Autodesk Inventor part; units mm, degrees
ref_plane "YZ Plane" through (0, 0, 0) normal (1, 0, 0) x (0, 1, 0)
ref_plane "XZ Plane" through (0, 0, 0) normal (0, 1, 0) x (-1, 0, 0)
ref_plane "XY Plane" through (0, 0, 0) normal (0, 0, 1) x (1, 0, 0)
sketch "Sketch1" plane through (0, 0, 0) normal (0, 1, 0) x (-1, 0, 0)
  line L0 (29.21, 0) -> (29.21, 12.8)
  line L1 (29.21, 12.8) -> (0, 12.8)
  line L2 (29.21, 12.8) -> (13.21, 12.8)
  circle A0 centre (3.3025, 9.6) radius 1.5
  circle A1 centre (9.9075, 9.6) radius 1.5
  line L3 (0, 12.8) -> (0, 0)
  line L4 (0, 0) -> (29.21, 0)
  dimension "d0" = 12.8
  dimension "d1" = 16
  dimension "d4" = 3
  dimension "d5" = 3
extrude "Extrusion1" add sketch "Sketch1" along normal blind 3
sketch "Sketch2" plane through (0, 3, 0) normal (0, 1, 0) x (1, 0, 0)
  line L0 (0, 0) -> (-29.21, 0)
  line L1 (-29.21, -12.8) -> (0, -12.8)
  line L2 (-29.21, 0) -> (-26.21, 0)
  line L3 (-26.21, 0) -> (-26.21, -12.8)
  line L4 (-26.21, -12.8) -> (-29.21, -12.8)
  line L5 (-29.21, -12.8) -> (-29.21, 0)
  dimension "d8" = 3
extrude "Extrusion2" add sketch "Sketch2" along normal blind 29.2
sketch "Sketch3" plane through (-29.21, 0, 0) normal (-1, 0, 0) x (0, 0, 1)
  line L0 (12.8, 0) -> (12.8, 32.2)
  line L1 (12.8, 16.1) -> (0, 16.1)
  line L2 (0, 0) -> (0, 32.2)
  line L3 (6.4, 27.2) -> (12.3, 27.2)
  line L4 (12.3, 27.2) -> (12.3, 5)
  line L5 (12.3, 5) -> (0.5, 5)
  line L6 (0.5, 5) -> (0.5, 27.2)
  line L7 (0.5, 27.2) -> (6.4, 27.2)
  line L8 (0, 0) -> (12.8, 0)
  circle A0 centre (6.4, 2.5) radius 0.5
  line L9 (0, 32.2) -> (12.8, 32.2)
  circle A1 centre (6.4, 29.7) radius 0.5
  dimension "d12" = 5.9
  dimension "d13" = 11.8
  dimension "d14" = 1
  dimension "d15" = 1
extrude "Extrusion3" cut sketch "Sketch3" against normal blind 3 contours L4 L5 L6 L1 | L1 L6 L7 L3 L4 | A0 | A1
sketch "Эскиз5" plane through (0, 0, 0) normal (0, 0, -1) x (-1, 0, 0)
  line L0 (29.21, 0) -> (0, 0)
  line L1 (26.21, 32.2) -> (29.21, 32.2)
  line L2 (0, 0) -> (29.21, 0)
  line L3 (29.21, 0) -> (29.21, 32.2)
  line L4 (29.21, 32.2) -> (0, 32.2)
  line L5 (0, 32.2) -> (0, 0)
extrude "Выдавливание4" add sketch "Эскиз5" along normal blind 3
chamfer "Фаска1" distance 15 angle 45 1 edges at (0, 32.2, -1.5)
fillet "Сопряжение3" radius 3 2 edges at (0, 1.5, 12.8) (-27.71, 32.2, 12.8)
Verification items for the finished model (mm, model axes). A direction names the side the tool comes from. Round coordinates to 2 decimals unless told otherwise and drop trailing zeros. Order: outer loops, then holes, each group sorted by start corner. A loop starts at its lowest first (then second) coordinate and runs counter-clockwise, first axis right, second up. Notation, with made-up numbers: (-5, 56) - (36, 56) arc R13 cw to (36, 72) - close; hole circle Ø9 at (-30.5, -28). An arc over 180 degrees is marked (long way). Use CSV: the item, a comma, the result in double quotes. Start each with the question number.
1) Thickness scan on L1, parallel to Y at x = -28.4, z = 6.4; L2, parallel to Y at x = -27, z = 8.75; L3, parallel to Z at x = -8.25, y = 4. Record the ranges inside material, lowest first.
2) Go/stop test with flat-tipped pins: P1, Ø2, axis at x = -20, y = 9.5, coming from the +Z side; P2, Ø1.8, axis at x = -9.91, z = 9.6, coming from the +Y side; P3, Ø1, axis at y = 18, z = -1, coming from the +X side. Record where each tip stops, or that it passes through.
3) Section check A-A, the plane y = 23. Record the cut outline in (x, z), plus the area to 3 significant figures.
4) Access from +Z, -Z, +X, -X, +Y, -Y to the whole of each face (thin tool, end or side, straight path). Record for faces 1 (the flat face through (-26.21, 20.8, 0.2)), 2 (the flat face through (-28, 5, 6)), 3 (the flat face through (-26.21, 2.5, 6.4)), 4 (the cylindrical face through (-27.69, 31.34, 11.9)).
5) Mould release check, pull along Y, two halves, no side actions. Record for faces 5 (the flat face through (-14, 16, -3)), 6 (the cylindrical face through (-27.731, 2.65, 6.877)), 7 (the flat face through (-15, 0, 5)), 8 (the flat face through (-28, 16, 12.3)): +Y half, -Y half, draft (parallel to the pull), parting line (faces both ways), or undercut.
6) Section check C-C, the plane y = 2.5. Record the cut outline in (x, z), plus the area to 3 significant figures.
7) Section check B-B, the plane z = 3. Record the cut outline in (x, y), plus the area to 3 significant figures.
8) Section check D-D, the plane x = -24.75. Record the cut outline in (y, z), plus the area to 3 significant figures.
Answers:
1,L1,"y = 0 to 2, 3 to 5, 27.2 to 29.2, 30.2 to 32.2"
1,L2,"y = 0 to 5, 27.2 to 32.2"
1,L3,"z = -3 to 0"
2,P1,"stops at z = 0"
2,P2,"passes through"
2,P3,"stops at x = -0.3"
3,outline,"(-29.21, -3) - (-5.8, -3) - (-5.8, 0) - (-26.21, 0) - (-26.21, 0.5) - (-29.21, 0.5) - close; (-29.21, 12.3) - (-26.21, 12.3) - (-26.21, 12.8) - (-29.21, 12.8) - close"
3,area,"73.2 mm²"
4,face 1,"+Z, +X, +Y"
4,face 2,"+X, -X"
4,face 3,"-X"
4,face 4,"+Z, +X, -X, +Y"
5,face 5,"draft"
5,face 6,"undercut"
5,face 7,"-Y half"
5,face 8,"undercut"
6,outline,"(-29.21, -3) - (0, -3) - (0, 9.8) arc R3 ccw to (-3, 12.8) - (-29.21, 12.8) - (-29.21, 6.9) - (-26.21, 6.9) - (-26.21, 5.9) - (-29.21, 5.9) - close; hole circle Ø3 at (-9.91, 9.6); hole circle Ø3 at (-3.3, 9.6)"
6,area,"442 mm²"
7,outline,"(-29.21, 0) - (0, 0) - (0, 3) - (-26.21, 3) - (-26.21, 5) - (-29.21, 5) - close; (-29.21, 27.2) - (-26.21, 27.2) - (-26.21, 32.2) - (-29.21, 32.2) - close"
7,area,"109 mm²"
8,outline,"(0, -3) - (32.2, -3) - (32.2, 0) - (3, 0) - (3, 12.8) - (0, 12.8) - close"
8,area,"135 mm²"
